Part model, mm, in its own coordinate system. Face numbers are marked on the shaded views. Give positions to 0.01 mm unless a question says otherwise; leave off trailing zeros. Write each loop counter-clockwise with the first axis right and the second up, starting at its lowest first coordinate (ties: lowest second). Pieces come first, ordered by that corner, then holes. Notation, with made-up numbers: M -10,77 L 1,77 A4 ccw 1,83 Z; hole C 59,75 d10. An arc over 180 degrees is marked long. Use CSV: the item, a comma, the result in double quotes. Start each with the question number.
Item 1: Cut at B-B (y = 9). List the corners of the cut face in (x, z), then the cut area to 3 significant figures.
Item 2: Cut at C-C (x = 13.5). List the corners of the cut face in (y, z).
Item 3: Pin check, flat tip, straight feed: pin 1 (12 mm diameter, centred on x = 12.5, z = -9, fed in from -Y). Stop position of the tip, or through.
Item 4: Cut at D-D (y = 17.5). List the corners of the cut face in (x, z), then the cut area to 3 significant figures.
Item 5: Mould opens along X. For the marked faces 1, 2 and 3 say: released by +X, released by -X, zero draft, split by the parting line, or undercut.
Item 6: Drill centre lines: line 1 (Z direction, x = 12, y = 6.5); line 2 (X direction, y = 2, z = -7.25); line 3 (X direction, y = 8, z = -8.5). Where is each one in solid material? Low to high. Write a range as [from, to].
Item 7: Cut at A-A (z = -9). List the corners of the cut face in (x, y), then the cut area to 3 significant figures.
from build123d import *

# Parameters (mm, degrees)
SKETCH_1_W          = 34
SKETCH_1_H          = 30
EXTRUDE_1_DEPTH     = 22
SKETCH_2_R          = 2.15
CUT_EXTRUDE_1_DEPTH = 23
SKETCH_3_R          = 4
CUT_EXTRUDE_2_DEPTH = 31


with BuildPart() as part:
    # 草图1 → 凸台-拉伸1 (new body)
    with BuildSketch(Plane(origin=(0, 0, 0), x_dir=(1, 0, 0), z_dir=(0, 1, 0))):
        Rectangle(SKETCH_1_W, SKETCH_1_H)
    extrude(amount=EXTRUDE_1_DEPTH)

    # 草图2 → 切除-拉伸1 (cut, through all)
    with BuildSketch(Plane(origin=(0, 22, 0), x_dir=(1, 0, 0), z_dir=(0, 1, 0))):
        with Locations((-12, 9)):
            Circle(SKETCH_2_R)
        with Locations((12, 9)):
            Circle(SKETCH_2_R)
        with Locations((12, -9)):
            Circle(SKETCH_2_R)
        with Locations((-12, -9)):
            Circle(SKETCH_2_R)
    extrude(amount=-CUT_EXTRUDE_1_DEPTH, mode=Mode.SUBTRACT)

    # 草图3 → 切除-拉伸2 (cut, through all)
    with BuildSketch(Plane.XY.offset(15)):
        with Locations((0, 11)):
            Circle(SKETCH_3_R)
    extrude(amount=-CUT_EXTRUDE_2_DEPTH, mode=Mode.SUBTRACT)


solid = part.part
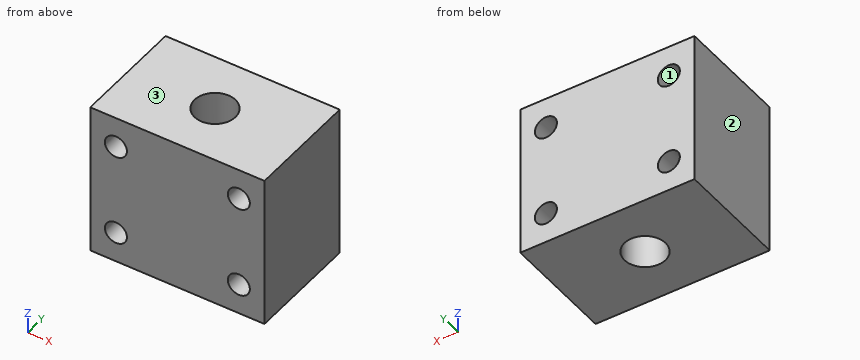
Worked answers:
1,outline,"M -17,-15 L -3.46,-15 L -3.46,15 L -17,15 Z; M 3.46,-15 L 17,-15 L 17,15 L 3.46,15 Z; hole C -12,-9 d4.3; hole C -12,9 d4.3; hole C 12,-9 d4.3; hole C 12,9 d4.3"
1,area,"754 mm^2"
2,outline,"M 0,-15 L 22,-15 L 22,-10.54 L 0,-10.54 Z; M 0,-7.46 L 22,-7.46 L 22,7.46 L 0,7.46 Z; M 0,10.54 L 22,10.54 L 22,15 L 0,15 Z"
3,pin 1,"stops at y = 0"
4,outline,"M -17,-15 L 17,-15 L 17,15 L -17,15 Z; hole C -12,-9 d4.3; hole C -12,9 d4.3; hole C 12,-9 d4.3; hole C 12,9 d4.3"
4,area,"962 mm^2"
5,face 1,"undercut"
5,face 2,"released by -X"
5,face 3,"zero draft"
6,line 1,"z = [-15, -11.15], [-6.85, 6.85], [11.15, 15]"
6,line 2,"x = [-17, -13.25], [-10.75, 10.75], [13.25, 17]"
6,line 3,"x = [-17, -14.09], [-9.91, -2.65], [2.65, 9.91], [14.09, 17]"
7,outline,"M -17,0 L -14.15,0 L -14.15,22 L -17,22 Z; M -9.85,0 L 9.85,0 L 9.85,22 L -9.85,22 Z; M 14.15,0 L 17,0 L 17,22 L 14.15,22 Z; hole C 0,11 d8"
7,area,"509 mm^2"
